Design review of the part built by this model. Coordinates are the model's own, in mm. A direction names the side the tool comes from. Coordinates: 2 decimals unless noted, no trailing zeros. Order: outer loops, then holes, each group sorted by start corner. A loop starts at its lowest first (then second) coordinate and runs counter-clockwise, first axis right, second up. Notation, with made-up numbers: (70.5, 53) -> (112.5, 53) arc R27 ccw to (112.5, 79) -> close; hole circle Ø1 at (-24, 19.25). An arc over 180 degrees is marked (long way). Write item = value, one per line.
```python
from build123d import *

# Parameters (mm, degrees)
SALIENTE_EXTRUIR1_DEPTH   = 230
SALIENTE_EXTRUIR1_2_DEPTH = 230
SALIENTE_EXTRUIR1_3_DEPTH = 230
SALIENTE_EXTRUIR1_4_DEPTH = 230
SALIENTE_EXTRUIR2_REACH   = 355.977
SALIENTE_EXTRUIR3_DEPTH   = 180
CROQUIS4_W                = 149.2
CROQUIS4_H                = 3.175
SALIENTE_EXTRUIR4_DEPTH   = 154.6
CROQUIS5_R                = 160
SALIENTE_EXTRUIR5_DEPTH   = 2
SALIENTE_EXTRUIR6_DEPTH   = 160
CROQUIS7_W                = 180
CROQUIS7_H                = 181.710341205
SALIENTE_EXTRUIR7_DEPTH   = 2
VACIADO1_START            = -150
VACIADO1_DEPTH            = 136
VACIADO1_START_2          = -14
VACIADO1_2_OUTLINE_R      = 148
VACIADO1_2_DEPTH          = 2
VACIADO1_START_3          = -12
VACIADO1_3_DEPTH          = 3.175
CROQUIS8_R                = 50
CORTAR_EXTRUIR1_DEPTH     = 14


# Read off the part's stored shape, not the designer's step: Vaciado1
with BuildPart() as part:
    # Croquis1 → Saliente-Extruir1 (new body)
    with BuildSketch(Plane(origin=(0, 0, 0), x_dir=(1, 0, 0), z_dir=(0, 1, 0))):
        Polygon((0, 0), (25.4, 0), (25.4, -3.175), (3.175, -3.175), (3.175, -25.4), (0, -25.4), align=None)
    extrude(amount=SALIENTE_EXTRUIR1_DEPTH)

    # Saliente-Extruir2: up to this face of the body (flat: up to its plane)
    saliente_extruir2_end = Plane(part.part.faces().sort_by_distance((12.7, 115, 0))[0])
    # Croquis2 → Saliente-Extruir2 (add, up to the picked face)
    with BuildSketch(Plane.XY.offset(200), mode=Mode.PRIVATE) as saliente_extruir2_sk1:
        Polygon((25.4, 230), (0, 230), (0, 204.6), (3.175, 204.6), (3.175, 226.825), (25.4, 226.825), align=None)
    saliente_extruir2_tool1 = split(extrude(saliente_extruir2_sk1.sketch, amount=-SALIENTE_EXTRUIR2_REACH, mode=Mode.PRIVATE), bisect_by=saliente_extruir2_end, keep=Keep.BOTH, mode=Mode.PRIVATE)
    # Croquis2 → Saliente-Extruir2 (add, up to the picked face)
    with BuildSketch(Plane.XY.offset(200), mode=Mode.PRIVATE) as saliente_extruir2_sk2:
        Polygon((176.825, 204.6), (180, 204.6), (180, 230), (154.6, 230), (154.6, 226.825), (176.825, 226.825), align=None)
    saliente_extruir2_tool2 = split(extrude(saliente_extruir2_sk2.sketch, amount=-SALIENTE_EXTRUIR2_REACH, mode=Mode.PRIVATE), bisect_by=saliente_extruir2_end, keep=Keep.BOTH, mode=Mode.PRIVATE)
    # Croquis2 → Saliente-Extruir2 (add, up to the picked face)
    with BuildSketch(Plane.XY.offset(200), mode=Mode.PRIVATE) as saliente_extruir2_sk3:
        Polygon((154.6, 0), (180, 0), (180, 25.4), (176.825, 25.4), (176.825, 3.175), (154.6, 3.175), align=None)
    saliente_extruir2_tool3 = split(extrude(saliente_extruir2_sk3.sketch, amount=-SALIENTE_EXTRUIR2_REACH, mode=Mode.PRIVATE), bisect_by=saliente_extruir2_end, keep=Keep.BOTH, mode=Mode.PRIVATE)
    # Croquis2 → Saliente-Extruir2 (add, up to the picked face)
    with BuildSketch(Plane.XY.offset(200), mode=Mode.PRIVATE) as saliente_extruir2_sk4:
        Polygon((3.175, 25.4), (0, 25.4), (0, 0), (25.4, 0), (25.4, 3.175), (3.175, 3.175), align=None)
    saliente_extruir2_tool4 = split(extrude(saliente_extruir2_sk4.sketch, amount=-SALIENTE_EXTRUIR2_REACH, mode=Mode.PRIVATE), bisect_by=saliente_extruir2_end, keep=Keep.BOTH, mode=Mode.PRIVATE)


with BuildPart() as body_2:
    # Croquis1 → Saliente-Extruir1 2 (new body)
    with BuildSketch(Plane(origin=(0, 0, 0), x_dir=(1, 0, 0), z_dir=(0, 1, 0))):
        Polygon((176.825, -25.4), (180, -25.4), (180, 0), (154.6, 0), (154.6, -3.175), (176.825, -3.175), align=None)
    extrude(amount=SALIENTE_EXTRUIR1_2_DEPTH)


with BuildPart() as body_3:
    # Croquis1 → Saliente-Extruir1 3 (new body)
    with BuildSketch(Plane(origin=(0, 0, 0), x_dir=(1, 0, 0), z_dir=(0, 1, 0))):
        Polygon((180, -200), (154.6, -200), (154.6, -196.825), (176.825, -196.825), (176.825, -174.6), (180, -174.6), align=None)
    extrude(amount=SALIENTE_EXTRUIR1_3_DEPTH)


with BuildPart() as body_4:
    # Croquis1 → Saliente-Extruir1 4 (new body)
    with BuildSketch(Plane(origin=(0, 0, 0), x_dir=(1, 0, 0), z_dir=(0, 1, 0))):
        Polygon((3.175, -174.6), (0, -174.6), (0, -200), (25.4, -200), (25.4, -196.825), (3.175, -196.825), align=None)
    extrude(amount=SALIENTE_EXTRUIR1_4_DEPTH)


with BuildPart() as part_1:
    add(part.part)

    add(body_2.part)  # Saliente-Extruir2 merges body 2

    add(body_3.part)  # Saliente-Extruir2 merges body 3

    add(body_4.part)  # Saliente-Extruir2 merges body 4
    add(saliente_extruir2_tool1.solids().sort_by(Axis((12.7, 229.64079, 200), (0, 0, -1)))[0])
    add(saliente_extruir2_tool2.solids().sort_by(Axis((178.4125, 204.95921, 200), (0, 0, -1)))[0])
    add(saliente_extruir2_tool3.solids().sort_by(Axis((167.3, 0.35921, 200), (0, 0, -1)))[0])
    add(saliente_extruir2_tool4.solids().sort_by(Axis((1.5875, 25.04079, 200), (0, 0, -1)))[0])

    # Croquis3 → Saliente-Extruir3 (add)
    with BuildSketch(Plane.ZY):
        Polygon((0, 0), (25.4, 0), (25.4, 3.175), (3.175, 3.175), (3.175, 25.4), (0, 25.4), align=None)
        Polygon((196.825, 25.4), (200, 25.4), (200, 0), (174.6, 0), (174.6, 3.175), (196.825, 3.175), align=None)
        Polygon((200, 230), (174.6, 230), (174.6, 226.825), (196.825, 226.825), (196.825, 204.6), (200, 204.6), align=None)
        Polygon((3.175, 204.6), (0, 204.6), (0, 230), (25.4, 230), (25.4, 226.825), (3.175, 226.825), align=None)
    extrude(amount=-SALIENTE_EXTRUIR3_DEPTH)

    # Croquis4 → Saliente-Extruir4 (add)
    with BuildSketch(Plane(origin=(180, 0, 0), x_dir=(0, 0, -1), z_dir=(1, 0, 0))):
        with Locations((-100, 228.4125)):
            Rectangle(CROQUIS4_W, CROQUIS4_H)
    extrude(amount=-SALIENTE_EXTRUIR4_DEPTH)

    # Croquis5 → Saliente-Extruir5 (add)
    with BuildSketch(Plane.ZY):
        with Locations(Location((100, 290, 0), (0, 0, 231.317812547))):
            Circle(CROQUIS5_R)
    extrude(amount=SALIENTE_EXTRUIR5_DEPTH)

    # Croquis6 → Saliente-Extruir6 (add)
    with BuildSketch(Plane.ZY.offset(2)):
        with BuildLine():
            Line((356.150943647, 460), (214.440602442, 460))
            Line((214.440602442, 460), (214.440602442, 423.899354359))
            ThreePointArc((214.440602442, 423.899354359), (159.743155313, 449.947233376), (100, 460))
            ThreePointArc((100, 460), (-76.81003198, 283.18996802), (100, 106.379936039))
            ThreePointArc((100, 106.379936039), (269.093013095, 152.354443037), (356.150943647, 304.430144907))
            Line((356.150943647, 304.430144907), (356.150943647, 460))
        make_face()
    extrude(amount=SALIENTE_EXTRUIR6_DEPTH)

    # Croquis7 → Saliente-Extruir7 (add)
    with BuildSketch(Plane(origin=(0, 460, 0), x_dir=(1, 0, 0), z_dir=(0, 1, 0))):
        with Locations((-82, -285.295773045)):
            Rectangle(CROQUIS7_W, CROQUIS7_H)
    extrude(amount=-SALIENTE_EXTRUIR7_DEPTH)

    # Vaciado1 outline → Vaciado1 (cut)
    with BuildSketch(Plane.YZ.offset(VACIADO1_START)):
        with BuildLine():
            Line((460, 344.150943647), (305.204872044, 344.150943647))
            ThreePointArc((305.204872044, 344.150943647), (161.38343221, 261.150196169), (118.381694611, 100.761352414))
            ThreePointArc((118.381694611, 100.761352414), (282.726065317, -64.809379089), (447.999915945, 99.833548521))
            ThreePointArc((447.999915945, 99.833548521), (434.67491503, 167.171792789), (400.045404599, 226.440602442))
            Line((400.045404599, 226.440602442), (460, 226.440602442))
            Line((460, 226.440602442), (460, 344.150943647))
        make_face()
    extrude(amount=VACIADO1_DEPTH, mode=Mode.SUBTRACT)

    # Vaciado1 2 outline → Vaciado1 2 (cut)
    with BuildSketch(Plane.YZ.offset(VACIADO1_START_2)):
        with Locations((290, 100)):
            Circle(VACIADO1_2_OUTLINE_R)
    extrude(amount=VACIADO1_2_DEPTH, mode=Mode.SUBTRACT)

    # Vaciado1 3 outline → Vaciado1 3 (cut)
    with BuildSketch(Plane.YZ.offset(VACIADO1_START_3)):
        with BuildLine():
            Line((169.981501426, 186.6), (216.6, 186.6))
            Line((216.6, 186.6), (216.6, 13.4))
            Line((216.6, 13.4), (169.981501426, 13.4))
            ThreePointArc((169.981501426, 13.4), (170.490801521, 12.698502424), (171.004201755, 12))
            Line((171.004201755, 12), (218, 12))
            Line((218, 12), (218, 188))
            Line((218, 188), (171.004201755, 188))
            ThreePointArc((171.004201755, 188), (170.490801521, 187.301497576), (169.981501426, 186.6))
        make_face()
    extrude(amount=VACIADO1_3_DEPTH, mode=Mode.SUBTRACT)

    # Croquis8 → Cortar-Extruir1 (cut)
    with BuildSketch(Plane.ZY.offset(162)):
        with Locations((100, 290)):
            Circle(CROQUIS8_R)
    extrude(amount=-CORTAR_EXTRUIR1_DEPTH, mode=Mode.SUBTRACT)


solid = part_1.part
```
(1) The part is to be moulded in two halves that separate along Y. For faces 4 (the flat face through (-96, 458, 359)), 5 (the cylindrical face through (-80.88, 287.078, -76.767)), 6 (the flat face through (9, 113, 200)), say which applies: released by +Y, released by -Y, zero draft, split by the parting line, or undercut.
Report:
face_4 = undercut
face_5 = split by the parting line
face_6 = zero draft
(2) For L1, parallel to Y at x = -155, z = 100; L2, parallel to X at y = 297, z = 238; L3, parallel to X at y = 128, z = 131.5, list the stretches that pass through material, from the lowest coordinate up.
Report:
L1 = 106.38 to 240, 340 to 460
L2 = -162 to -150, -12 to 0
L3 = -162 to -150, -14 to -2
(3) Insertion check: pin 1 (10 mm diameter, centred on y = 368.5, z = 71.5, fed in from -X); pin 2 (1 mm diameter, centred on x = 83.5, z = 1.5, fed in from -Y); pin 3 (10 mm diameter, centred on y = 134.5, z = 234, fed in from +X); pin 4 (5 mm diameter, centred on x = 30.5, z = 172, fed in from -Y) (3 decimals). Each pin has a flat end and moves straight along its axis. Give the tip position at first contact, or say it passes through.
Report:
pin_1 = -162
pin_2 = 0
pin_3 = -2
pin_4 = 226.825
(4) We need section A-A (x = 58). Write out the cut boundary in (y, z) (3 decimals), and give its area (3 significant figures).
Report:
outline = (0, 0) -> (25.4, 0) -> (25.4, 3.175) -> (3.175, 3.175) -> (3.175, 25.4) -> (0, 25.4) -> close; (0, 174.6) -> (3.175, 174.6) -> (3.175, 196.825) -> (25.4, 196.825) -> (25.4, 200) -> (0, 200) -> close; (204.6, 0) -> (230, 0) -> (230, 200) -> (204.6, 200) -> (204.6, 196.825) -> (226.825, 196.825) -> (226.825, 3.175) -> (204.6, 3.175) -> close
area = 1,080 mm²
(5) We need section C-C (y = 290). Write out the cut boundary in (x, z), and give its area (3 significant figures).
Report:
outline = (-162, -76.68) -> (-2, -76.68) -> (-2, -60) -> (0, -60) -> (0, 260) -> (-2, 260) -> (-2, 353.83) -> (-162, 353.83) -> (-162, 150) -> (-150, 150) -> (-150, 341.6) -> (-14, 341.6) -> (-14, 248) -> (-12, 248) -> (-12, -48) -> (-14, -48) -> (-14, -64.67) -> (-150, -64.67) -> (-150, 50) -> (-162, 50) -> close
area = 12,500 mm²
(6) For faces 1 (the flat face through (91, 226.825, 101)), 2 (the flat face through (9, 113, 0)), 3 (the flat face through (9, 0, 99)), list the 3-axis set-ups (+Z, -Z, +X, -X, +Y, -Y) from which the entire face can be reached by the end or side of a thin tool; tool diameter is ignored.
Report:
face_1 = none
face_2 = -Z, +X, +Y, -Y
face_3 = +Z, -Z, +X, -X, -Y
(7) We need section D-D (z = 43). Give the number of separate pieces and of enclosed holes in the cut face, and give its area (3 significant figures).
Report:
separate_pieces = 3
enclosed_holes = 1
area = 12,600 mm²
(8) We need section B-B (z = -7.5). Write out the cut boundary in (x, y), and give its area (3 significant figures).
Report:
outline = (-162, 142.81) -> (-2, 142.81) -> (-2, 171.49) -> (0, 171.49) -> (0, 408.51) -> (-2, 408.51) -> (-2, 423.57) -> (-162, 423.57) -> close; hole (-150, 158.27) -> (-14, 158.27) -> (-14, 188.28) -> (-12, 188.28) -> (-12, 391.72) -> (-14, 391.72) -> (-14, 408.11) -> (-150, 408.11) -> close
area = 11,000 mm²
